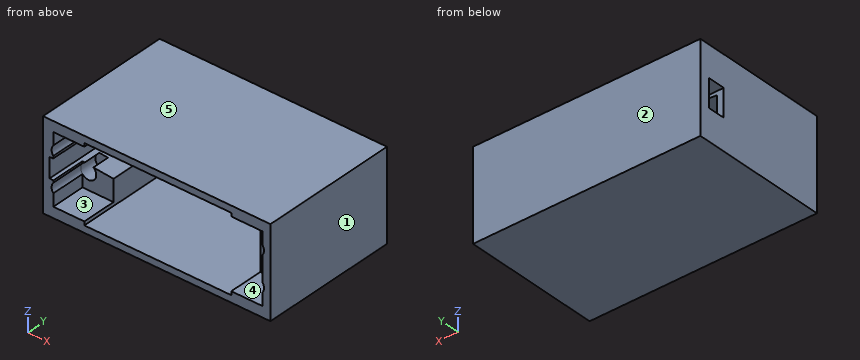
Solid Edge part; units mm, degrees
sketch "Sketch1" plane through (0, 0, 0) normal (0, -1, 0) x (1, 0, 0)
  line L0 (31.4924, 35.0939) -> (97.4924, 35.0939)
  line L1 (97.4924, 35.0939) -> (97.4924, 9.0939)
  line L2 (97.4924, 9.0939) -> (31.4924, 9.0939)
  line L3 (31.4924, 9.0939) -> (31.4924, 35.0939)
  dimension "D1" = 31.4924
  dimension "D2" = 97.4924
extrude "Protrusion1" add sketch "Sketch1" against normal blind 40
sketch "Sketch2" plane through (64.4924, 0, 22.0939) normal (0, -1, 0) x (1, 0, 0)
  line L0 (-31.0616, 2.8803) -> (-21, 3.7605)
  line L1 (-21, 3.7605) -> (-21, 11.0605)
  line L2 (-21, 11.0605) -> (21.64, 11.0605)
  line L3 (21.64, -11) -> (21.64, 11.0605)
  line L4 (-21, -11) -> (21.64, -11)
  line L5 (-21, -11) -> (-21, -3.7)
  line L6 (-21, -3.7) -> (-31.0616, -2.8197)
  line L7 (-31.0616, -2.8197) -> (-31.0616, 2.8803)
extrude "ExtrudedCutout_4" cut sketch "Sketch2" against normal blind 37
sketch "Sketch3" plane through (31.4924, 20, 22.0939) normal (-1, 0, 0) x (0, -1, 0)
  line L0 (-17, -4) -> (-17, 4)
  line L1 (-17, 4) -> (-12, 4)
  line L2 (-12, 4) -> (-12, -4)
  line L3 (-12, -4) -> (-17, -4)
  dimension "D1" = 17
  dimension "D2" = 17
  dimension "D3" = 12
extrude "Cutout1" cut sketch "Sketch3" against normal up to next
sketch "Sketch4" plane through (64.4924, 0, 22.0939) normal (0, -1, 0) x (1, 0, 0)
  line L0 (-21, 10.0605) -> (-30, 10.0605)
  line L1 (-30, 10.0605) -> (-30, -9.9395)
  line L2 (-30, -9.9395) -> (-21, -9.9395)
  line L3 (-21, -9.9395) -> (-21, 10.0605)
  line L4 (21.64, 10.0605) -> (30.64, 10.0605)
  line L5 (30.64, 10.0605) -> (30.64, -9.9395)
  line L6 (30.64, -9.9395) -> (21.64, -9.9395)
  line L7 (21.64, -9.9395) -> (21.64, 10.0605)
  dimension "D1" = 30.64
  dimension "D2" = 21
  dimension "D3" = 30
  dimension "D4" = 21.64
extrude "ExtrudedCutout_6" cut sketch "Sketch4" against normal blind 10
sketch "Sketch5" plane through (91.2324, 10, 21.645) normal (0, -1, 0) x (1, 0, 0)
  circle A0 centre (2.15, 5.5095) radius 2.25
  circle A1 centre (-54.99, 5.5095) radius 2.25
  circle A2 centre (-54.99, -4.4905) radius 2.25
  circle A3 centre (2.15, -4.4905) radius 2.25
  dimension "D1" = 54.99
  dimension "D2" = 2.15
  dimension "D3" = 54.99
extrude "ExtrudedCutout_7" cut sketch "Sketch5" against normal blind 5
sketch "Sketch6" plane through (64.4924, 0, 22.0939) normal (0, -1, 0) x (1, 0, 0)
  circle A0 centre (28.89, 5.0605) radius 2.25
  circle A1 centre (28.89, -4.9395) radius 2.25
  circle A2 centre (-28.25, 5.0605) radius 2.25
  circle A3 centre (-28.25, -4.9395) radius 2.25
extrude "Cutout2" cut sketch "Sketch6" against normal up to next
Work out the finished part from the listing and answer in its coordinate system (mm). Face numbers are marked on the shaded views. A direction names the side the tool comes from. Round coordinates to 2 decimals unless told otherwise and drop trailing zeros. Write each loop counter-clockwise with the first axis right and the second up, starting at its lowest first coordinate (ties: lowest second). Pieces come first, ordered by that corner, then holes. Notation, with made-up numbers: (0, 77) -> (24, 77) arc R27 cw to (24, 110) -> close; hole circle Ø1 at (11.25, 73). An arc over 180 degrees is marked (long way). Answer as CSV lines item,"result". Start each with the question number.
(1) The mould has two halves that part along X. Classify the marked faces 1, 2 and 3: +X half, -X half, draft (parallel to the pull), parting line (faces both ways), or undercut.
(2) Each of these flat-tipped pins is pushed along its axis until it touches: pin 1 (2 mm diameter, centred on x = 84.5, z = 13, fed in from -Y); pin 2 (3.5 mm diameter, centred on x = 37.5, z = 27, fed in from -Y). Where does it stop, or does it pass through?
(3) Find the intervals of material crossed by probe 1 along X at (y, z) = (34, 16.75); probe 2 along Z at (x, y) = (40, 4.5); probe 3 along Z at (x, y) = (66, 35), in increasing order.
(4) The part is cut by section C-C, the plane x = 56.5. Give the vertices of the cut face in (y, z), then the cut area to 3 significant figures.
(5) The part is cut by section A-A, the plane y = 19. Give the vertices of the cut face in (x, z).
(6) The part is cut by section B-B, the plane z = 24.25. Give the vertices of the cut face in (x, y), then the cut area to 3 significant figures.
(7) A tool of negligible diameter and unlimited length cuts with its end or side. For the marked faces 4 and 5, from which of +Z, -Z, +X, -X, +Y, -Y can it reach the whole face along a straight path? Write none if from no direction.
(8) The part is cut by section D-D, the plane y = 14. Give the vertices of the cut face in (x, z).
Output values:
1,face 1,"+X half"
1,face 2,"draft"
1,face 3,"undercut"
2,pin 1,"stops at y = 37"
2,pin 2,"stops at y = 10"
3,probe 1,"x = 31.49 to 43.49, 86.13 to 97.49"
3,probe 2,"z = 9.09 to 12.15, 32.15 to 35.09"
3,probe 3,"z = 9.09 to 11.09, 33.15 to 35.09"
4,outline,"(0, 9.09) -> (40, 9.09) -> (40, 35.09) -> (0, 35.09) -> (0, 33.15) -> (37, 33.15) -> (37, 11.09) -> (0, 11.09) -> close"
4,area,"224 mm²"
5,outline,"(31.49, 9.09) -> (97.49, 9.09) -> (97.49, 35.09) -> (31.49, 35.09) -> close; hole (33.43, 19.27) -> (43.49, 18.39) -> (43.49, 11.09) -> (86.13, 11.09) -> (86.13, 33.15) -> (43.49, 33.15) -> (43.49, 25.85) -> (33.43, 24.97) -> close"
6,outline,"(31.49, 0) -> (33.43, 0) -> (33.43, 32) -> (31.49, 32) -> close; (31.49, 37) -> (86.13, 37) -> (86.13, 10) -> (95.13, 10) -> (95.13, 0) -> (97.49, 0) -> (97.49, 40) -> (31.49, 40) -> close"
6,area,"590 mm²"
7,face 4,"-Y"
7,face 5,"+Z, +X, -X, +Y, -Y"
8,outline,"(31.49, 9.09) -> (97.49, 9.09) -> (97.49, 35.09) -> (31.49, 35.09) -> close; hole (33.43, 19.27) -> (35.15, 19.12) arc R2.25 ccw (long way) to (37.66, 18.9) -> (43.49, 18.39) -> (43.49, 11.09) -> (86.13, 11.09) -> (86.13, 33.15) -> (43.49, 33.15) -> (43.49, 25.85) -> (37.57, 25.34) arc R2.25 ccw (long way) to (35.25, 25.13) -> (33.43, 24.97) -> close; hole circle Ø4.5 at (93.38, 17.15); hole circle Ø4.5 at (93.38, 27.15)"
